Can you work these out from the model? Positions are in its coordinate system, mm. Face numbers are marked on the shaded views. A direction names the side the tool comes from. Give positions to 0.01 mm unless a question says otherwise; leave off trailing zeros. Loops run counter-clockwise (first coordinate to the right, second up) from the corner with the lowest first, then second, coordinate; pieces in that order, holes last. Notation, with made-up numbers: (-20.5, 61.25) - (2.5, 61.25) arc R11 ccw to (2.5, 74.25) - close; hole circle Ø11 at (66, -25.75). An arc over 180 degrees is marked (long way). Answer as a JSON object with one key per item and string values.
```python
from build123d import *

# Parameters (mm, degrees)
SALIENTE_EXTRUIR1_DEPTH    = 8
SALIENTE_EXTRUIR2_DEPTH    = 12
CORTAR_EXTRUIR3_DEPTH      = 173.609385608
CORTAR_EXTRUIR3_DEPTH_BACK = 173.609385608
CROQUIS7_R                 = 25
CROQUIS7_R_2               = 1.75
SALIENTE_EXTRUIR4_START    = -3
SALIENTE_EXTRUIR4_DEPTH    = 3
CROQUIS10_R                = 1.6
CORTAR_EXTRUIR4_DEPTH      = 173.609385608


with BuildPart() as part:
    # Croquis1 → Saliente-Extruir1 (new body)
    with BuildSketch(Plane(origin=(0, 0, 0), x_dir=(1, 0, 0), z_dir=(0, 1, 0))):
        with BuildLine():
            Line((-71.345800689, 92.236983213), (-40.311288741, 20))
            ThreePointArc((-40.311288741, 20), (-45, 0), (-40.311288741, -20))
            Line((-40.311288741, -20), (-71.345800689, -92.236983213))
            ThreePointArc((-71.345800689, -92.236983213), (-44.837742086, -152.483425118), (13.414371956, -121.840283261))
            Line((13.414371956, -121.840283261), (43.414371956, -11.840283261))
            ThreePointArc((43.414371956, -11.840283261), (45, 0), (43.414371956, 11.840283261))
            Line((43.414371956, 11.840283261), (13.414371956, 121.840283261))
            ThreePointArc((13.414371956, 121.840283261), (-44.837742086, 152.483425118), (-71.345800689, 92.236983213))
        make_face()
    extrude(amount=SALIENTE_EXTRUIR1_DEPTH)

    # Croquis6 → Saliente-Extruir2 (add)
    with BuildSketch(Plane(origin=(0, 8, 0), x_dir=(1, 0, 0), z_dir=(0, 1, 0))):
        with BuildLine():
            Line((-39.280821918, 2.125330436), (-25.821917808, 19.73521119))
            ThreePointArc((-25.821917808, 19.73521119), (-16.25, 28.145825623), (-4.180235335, 32.230042391))
            Line((-4.180235335, 32.230042391), (17.79982081, 35.08085488))
            ThreePointArc((17.79982081, 35.08085488), (20, 34.641016151), (21.481001108, 32.955524444))
            Line((21.481001108, 32.955524444), (30.002153144, 12.494831201))
            ThreePointArc((30.002153144, 12.494831201), (32.5, 0), (30.002153144, -12.494831201))
            Line((30.002153144, -12.494831201), (21.481001108, -32.955524444))
            ThreePointArc((21.481001108, -32.955524444), (20, -34.641016151), (17.79982081, -35.08085488))
            Line((17.79982081, -35.08085488), (-4.180235335, -32.230042391))
            ThreePointArc((-4.180235335, -32.230042391), (-16.25, -28.145825623), (-25.821917808, -19.73521119))
            Line((-25.821917808, -19.73521119), (-39.280821918, -2.125330436))
            ThreePointArc((-39.280821918, -2.125330436), (-40, 0), (-39.280821918, 2.125330436))
        make_face()
        with BuildLine():
            Line((-69.280821918, -107.874669564), (-55.821917808, -90.26478881))
            ThreePointArc((-55.821917808, -90.26478881), (-46.25, -81.854174377), (-34.180235335, -77.769957609))
            Line((-34.180235335, -77.769957609), (-12.20017919, -74.91914512))
            ThreePointArc((-12.20017919, -74.91914512), (-10, -75.358983849), (-8.518998892, -77.044475556))
            Line((-8.518998892, -77.044475556), (0.002153144, -97.505168799))
            ThreePointArc((0.002153144, -97.505168799), (2.5, -110), (0.002153144, -122.494831201))
            Line((0.002153144, -122.494831201), (-8.518998892, -142.955524444))
            ThreePointArc((-8.518998892, -142.955524444), (-10, -144.641016151), (-12.20017919, -145.08085488))
            Line((-12.20017919, -145.08085488), (-34.180235335, -142.230042391))
            ThreePointArc((-34.180235335, -142.230042391), (-46.25, -138.145825623), (-55.821917808, -129.73521119))
            Line((-55.821917808, -129.73521119), (-69.280821918, -112.125330436))
            ThreePointArc((-69.280821918, -112.125330436), (-70, -110), (-69.280821918, -107.874669564))
        make_face()
        with BuildLine():
            Line((-69.280821918, 107.874669564), (-55.821917808, 90.26478881))
            ThreePointArc((-55.821917808, 90.26478881), (-46.25, 81.854174377), (-34.180235335, 77.769957609))
            Line((-34.180235335, 77.769957609), (-12.20017919, 74.91914512))
            ThreePointArc((-12.20017919, 74.91914512), (-10, 75.358983849), (-8.518998892, 77.044475556))
            Line((-8.518998892, 77.044475556), (0.002153144, 97.505168799))
            ThreePointArc((0.002153144, 97.505168799), (2.5, 110), (0.002153144, 122.494831201))
            Line((0.002153144, 122.494831201), (-8.518998892, 142.955524444))
            ThreePointArc((-8.518998892, 142.955524444), (-10, 144.641016151), (-12.20017919, 145.08085488))
            Line((-12.20017919, 145.08085488), (-34.180235335, 142.230042391))
            ThreePointArc((-34.180235335, 142.230042391), (-46.25, 138.145825623), (-55.821917808, 129.73521119))
            Line((-55.821917808, 129.73521119), (-69.280821918, 112.125330436))
            ThreePointArc((-69.280821918, 112.125330436), (-70, 110), (-69.280821918, 107.874669564))
        make_face()
    extrude(amount=SALIENTE_EXTRUIR2_DEPTH)

    # Croquis7 → Cortar-Extruir3 (cut, two sides: drawn at the far end of the back side and taken through both)
    with BuildSketch(Plane(origin=(0, 8, 0), x_dir=(1, 0, 0), z_dir=(0, 1, 0)).offset(-CORTAR_EXTRUIR3_DEPTH_BACK)):
        with Locations(Location((0, 0, 0), (0, 0, 270))):
            Circle(CROQUIS7_R)
        with Locations(Location((-30, 110, 0), (0, 0, 270))):
            Circle(CROQUIS7_R)
        with Locations(Location((-30, -110, 0), (0, 0, 270))):
            Circle(CROQUIS7_R)
        with Locations(Location((-36.5, 0, 0), (0, 0, 270))):
            Circle(CROQUIS7_R_2)
        with Locations(Location((18.25, -31.609927238, 0), (0, 0, 270))):
            Circle(CROQUIS7_R_2)
        with Locations(Location((18.25, 31.609927238, 0), (0, 0, 270))):
            Circle(CROQUIS7_R_2)
        with Locations(Location((-11.75, 141.609927238, 0), (0, 0, 270))):
            Circle(CROQUIS7_R_2)
        with Locations(Location((-66.5, 110, 0), (0, 0, 270))):
            Circle(CROQUIS7_R_2)
        with Locations(Location((-11.75, 78.390072762, 0), (0, 0, 270))):
            Circle(CROQUIS7_R_2)
        with Locations(Location((-66.5, -110, 0), (0, 0, 270))):
            Circle(CROQUIS7_R_2)
        with Locations(Location((-11.75, -141.609927238, 0), (0, 0, 270))):
            Circle(CROQUIS7_R_2)
        with Locations(Location((-11.75, -78.390072762, 0), (0, 0, 270))):
            Circle(CROQUIS7_R_2)
    extrude(amount=CORTAR_EXTRUIR3_DEPTH + CORTAR_EXTRUIR3_DEPTH_BACK, mode=Mode.SUBTRACT)

    # Croquis9 → Saliente-Extruir4 (add)
    with BuildSketch(Plane.XZ.offset(SALIENTE_EXTRUIR4_START)):
        with BuildLine():
            Line((-2.867032155, 8.492482473), (-12.199873602, 21.821161383))
            ThreePointArc((-12.199873602, 21.821161383), (0, 25), (12.199873602, 21.821161383))
            Line((12.199873602, 21.821161383), (2.867032155, 8.492482473))
            ThreePointArc((2.867032155, 8.492482473), (0, 7), (-2.867032155, 8.492482473))
        make_face()
        with BuildLine():
            Line((8.492482473, 2.867032155), (21.821161383, 12.199873602))
            ThreePointArc((21.821161383, 12.199873602), (25, 0), (21.821161383, -12.199873602))
            Line((21.821161383, -12.199873602), (8.492482473, -2.867032155))
            ThreePointArc((8.492482473, -2.867032155), (7, 0), (8.492482473, 2.867032155))
        make_face()
        with BuildLine():
            Line((2.867032155, -8.492482473), (12.199873602, -21.821161383))
            ThreePointArc((12.199873602, -21.821161383), (0, -25), (-12.199873602, -21.821161383))
            Line((-12.199873602, -21.821161383), (-2.867032155, -8.492482473))
            ThreePointArc((-2.867032155, -8.492482473), (0, -7), (2.867032155, -8.492482473))
        make_face()
        with BuildLine():
            Line((-8.492482473, -2.867032155), (-21.821161383, -12.199873602))
            ThreePointArc((-21.821161383, -12.199873602), (-25, 0), (-21.821161383, 12.199873602))
            Line((-21.821161383, 12.199873602), (-8.492482473, 2.867032155))
            ThreePointArc((-8.492482473, 2.867032155), (-7, 0), (-8.492482473, -2.867032155))
        make_face()
    extrude(amount=SALIENTE_EXTRUIR4_DEPTH)

    # Croquis10 → Cortar-Extruir4 (cut, through all)
    with BuildSketch(Plane(origin=(0, 8, 0), x_dir=(1, 0, 0), z_dir=(0, 1, 0))):
        with Locations(Location((-10.5, 0, 0), (0, 0, 270))):
            Circle(CROQUIS10_R)
        with Locations(Location((0, -10.5, 0), (0, 0, 270))):
            Circle(CROQUIS10_R)
        with Locations(Location((10.5, 0, 0), (0, 0, 270))):
            Circle(CROQUIS10_R)
        with Locations(Location((0, 10.5, 0), (0, 0, 270))):
            Circle(CROQUIS10_R)
    extrude(amount=-CORTAR_EXTRUIR4_DEPTH, mode=Mode.SUBTRACT)


solid = part.part
```
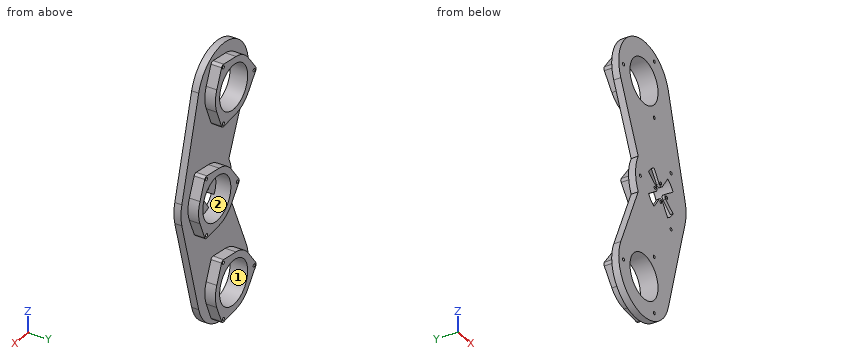
1) I need wall thicknesses on L1, parallel to X at y = 9.75, z = 0; L2, parallel to Z at x = 17, y = 10.75; L3, parallel to Z at x = -30, y = 19.25. Which ranges of each line are inside material? Lowest first, please.
Check sheet entries:
{"L1": "-40 to -38.25, -34.75 to -25, 25 to 32.5", "L2": "-34.98 to -32.83, -30.39 to -18.33, 18.33 to 30.39, 32.83 to 34.98", "L3": "-142.77 to -135, -85 to -77.23, -14.27 to 14.27, 77.23 to 85, 135 to 142.77"}
2) Imagine slicing it at B-B on z = -51. Write out the boundary of the cut face in (x, y), and give its area (3 significant figures).
Check sheet entries:
{"outline": "(-53.63, 0) - (32.73, 0) - (32.73, 8) - (-53.63, 8) - close", "area": "691 mm2"}
3) Imagine slicing it at A-A on z = 126. Write out the boundary of the cut face in (x, y), and give its area (3 significant figures).
Check sheet entries:
{"outline": "(-72.06, 0) - (-49.21, 0) - (-49.21, 20) - (-58.68, 20) - (-58.68, 8) - (-72.06, 8) - close; (-10.79, 0) - (12.06, 0) - (12.06, 8) - (-1.46, 8) - (-1.46, 20) - (-10.79, 20) - close", "area": "591 mm2"}
4) Which directions (+Z, -Z, +X, -X, +Y, -Y) give clear straight access to the entire face, cutting with the end or side of a thin tool? Please do the marked faces 1 and 2.
Check sheet entries:
{"face 1": "+Y, -Y", "face 2": "+Y"}
5) I'm going to push flat-ended pins straight in: P1, Ø4, axis at x = -53, y = 17.5, coming from the +Z side; P2, Ø2.5, axis at x = 10.5, z = 0, coming from the -Y side; P3, Ø8, axis at x = -16, y = 5, coming from the +Z side; P4, Ø2, axis at x = 15.5, z = 90, coming from the +Y side. Where does each tip first touch, or does it pass through?
Check sheet entries:
{"P1": "z = 134.8", "P2": "through", "P3": "z = 153.87", "P4": "y = 8"}
